Input: part model. Units: mm. Frame: model coordinates. A direction names the side the tool comes from. Round coordinates to 2 decimals unless told otherwise and drop trailing zeros. Loops run counter-clockwise (first coordinate to the right, second up) from the corner with the lowest first, then second, coordinate; pieces in that order, holes last.
(1) Line query: line 1 (Y direction, x = 6.5, z = 29); line 2 (X direction, y = 0, z = 7); line 3 (Y direction, x = 3.25, z = 6.5). Output: solid intervals per line, ascending.
(2) Cut plane A-A, the plane z = 26. Output: boundary loops of the cut face in (x, y).
(3) Access query for faces 5 (the face through (2.5, 0, 29)), 6 (the face through (0, 12.5, 24)). Directions: +Z, -Z, +X, -X, +Y, -Y. A direction counts if a zero-diameter tool reaches every point of the face in a straight line with its end or side. Return the directions, or none.
(4) Draft query along X for faces 1 (the face through (12.5, 6, 35)), 2 (the face through (0, -5, 0)), 3 (the face through (-0.867, -3.905, 6.096)), 4 (the face through (0.151, -0.678, 13.986)). Return one class per face: released by +X, released by -X, zero draft, split by the parting line, or undercut.
(5) First-contact query: pin 1 Ø7 at (x, y) = (0, 0) entering from -Z; pin 2 Ø11 at (y, z) = (-0.5, 28.5) entering from +X; pin 3 Ø1.5 at (y, z) = (3.5, 10) entering from +X. Flat tips, straight axial feed; report the tip coordinate or a pass-through.
from build123d import *

# Parameters (mm, degrees)
BOSS_EXTRUDE1_DEPTH             = 12.5
BOSS_EXTRUDE1_DEPTH_BACK        = 12.5
SKETCH4_R                       = 7
CUT_EXTRUDE1_DEPTH              = 10
F_8_0MM_DOWEL_HOLE1_D           = 8
F_8_0MM_DOWEL_HOLE1_DEPTH       = 12
F_8_0MM_DOWEL_HOLE1_CSINK_D     = 8.05
F_8_0MM_DOWEL_HOLE1_CSINK_ANGLE = 90
F_8_0MM_DOWEL_HOLE1_TIP         = 2.403442476


with BuildPart() as part:
    # Sketch2 → Loft1 section 0
    with BuildSketch(Plane.XY.offset(19)):
        with BuildLine():
            Line((-12.5, -12.5), (12.5, -12.5))
            Line((12.5, -12.5), (12.5, 12.5))
            Line((12.5, 12.5), (-12.5, 12.5))
            Line((-12.5, 12.5), (-12.5, -12.5))
        make_face()
    # Sketch1 → Loft1 section 1
    with BuildSketch(Plane.XY):
        with BuildLine():
            Line((-10, -10), (10, -10))
            Line((10, -10), (10, 10))
            Line((10, 10), (-10, 10))
            Line((-10, 10), (-10, -10))
        make_face()
    loft()

    # Sketch3 → Boss-Extrude1 (add, two sides: drawn at the far end of the back side and taken through both)
    with BuildSketch(Plane(origin=(0, 0, 0), x_dir=(0, 0, -1), z_dir=(1, 0, 0)).offset(-BOSS_EXTRUDE1_DEPTH_BACK)):
        with BuildLine():
            Line((-19, 12.5), (-29, 12.5))
            ThreePointArc((-29, 12.5), (-41.5, 0), (-29, -12.5))
            Line((-29, -12.5), (-19, -12.5))
            Line((-19, -12.5), (-19, 12.5))
        make_face()
    extrude(amount=BOSS_EXTRUDE1_DEPTH + BOSS_EXTRUDE1_DEPTH_BACK)

    # Sketch4 → Cut-Extrude1 (cut)
    with BuildSketch(Plane(origin=(12.5001, 0, 0), x_dir=(0, 0, -1), z_dir=(1, 0, 0))):
        with Locations((-29, 0)):
            Circle(SKETCH4_R)
    extrude(amount=-CUT_EXTRUDE1_DEPTH, mode=Mode.SUBTRACT)

    # Ø8.0mm Dowel Hole1
    with Locations(Plane(origin=(0, 0, 0), x_dir=(-1, 0, 0), z_dir=(0, 0, -1))):
        with Locations((0, 0)):
            CounterSinkHole(F_8_0MM_DOWEL_HOLE1_D / 2, F_8_0MM_DOWEL_HOLE1_CSINK_D / 2, depth=F_8_0MM_DOWEL_HOLE1_DEPTH, counter_sink_angle=F_8_0MM_DOWEL_HOLE1_CSINK_ANGLE)
            with Locations((0, 0, -(F_8_0MM_DOWEL_HOLE1_DEPTH + F_8_0MM_DOWEL_HOLE1_TIP / 2))):  # 118° drill point
                Cone(0, F_8_0MM_DOWEL_HOLE1_D / 2, F_8_0MM_DOWEL_HOLE1_TIP, mode=Mode.SUBTRACT)


solid = part.part
Reported:
1. line 1: y = -12.5 to -7, 7 to 12.5
1. line 2: x = -10.92 to -4, 4 to 10.92
1. line 3: y = -10.86 to -2.33, 2.33 to 10.86
2. outline: (-12.5, -12.5) - (12.5, -12.5) - (12.5, -6.32) - (2.5, -6.32) - (2.5, 6.32) - (12.5, 6.32) - (12.5, 12.5) - (-12.5, 12.5) - close
3. face 5: +X
3. face 6: +Z, -Z, +X, -X, +Y
4. face 1: released by +X
4. face 2: zero draft
4. face 3: undercut
4. face 4: undercut
5. pin 1: stops at z = 12.3
5. pin 2: stops at x = 2.5
5. pin 3: stops at x = 11.41
